Check sheet for the modelled part. Datum: model origin and axes. Units: mm. Round coordinates to 2 decimals unless told otherwise and drop trailing zeros. Write each loop counter-clockwise with the first axis right and the second up, starting at its lowest first coordinate (ties: lowest second). Pieces come first, ordered by that corner, then holes. Notation, with made-up numbers: (-18, 77) -> (11, 77) arc R32 cw to (11, 104) -> close; hole circle Ø1 at (29, 36.25). An arc over 180 degrees is marked (long way). Put each result on its own line as item: value. Start each with the question number.
from build123d import *

# Parameters (mm, degrees)
BOSS_EXTRUDE1_DEPTH     = 3.302
M3_CLEARANCE_HOLE1_D    = 3.4
SKETCH6_W               = 210.566
SKETCH6_H               = 3.302
BOSS_EXTRUDE3_DEPTH     = 1.62
SKETCH7_W               = 210.566
SKETCH7_H               = 3.302
BOSS_EXTRUDE4_DEPTH     = 5.18
M3_CLEARANCE_HOLE2_D    = 3.4
SKETCH21_R              = 20.32
CUT_EXTRUDE1_DEPTH      = 336.371396057
ADVANCEDHOLE1_OUTLINE_R = 1.6
ADVANCEDHOLE1_DEPTH     = 3.302
CUT_EXTRUDE2_REACH      = 337.371
SKETCH33_W              = 167.386
SKETCH33_H              = 21.59
FILLET1_R               = 6.35
CUT_EXTRUDE3_DEPTH      = 315.946962825
M5_CLEARANCE_HOLE1_D    = 5.5
M3_CLEARANCE_HOLE3_D    = 3.4
SKETCH40_W              = 22
SKETCH40_H              = 75
CUT_EXTRUDE4_DEPTH      = 315.946962825
FILLET2_R               = 3.81
FILLET3_R               = 2.032


# Read off the part's stored shape, not the designer's step: AdvancedHole1
with BuildPart() as part:
    # Sketch1 → Boss-Extrude1 (new body)
    with BuildSketch(Plane(origin=(0, 0, 0), x_dir=(1, 0, 0), z_dir=(0, 1, 0))):
        Polygon((105.283, -80.01), (105.283, 101.6), (-105.283, 101.6), (-105.283, -80.01), (-83.693, -80.01), (-83.693, -101.6), (83.693, -101.6), (83.693, -80.01), align=None)
    extrude(amount=BOSS_EXTRUDE1_DEPTH)

    # M3 Clearance Hole1 (through all)
    with Locations(Plane(origin=(0, 3.302, 0), x_dir=(1, 0, 0), z_dir=(0, 1, 0))):
        with Locations((-95.377, -54.61), (-95.377, 57.15), (95.377, 57.15), (95.377, -54.61)):
            Hole(M3_CLEARANCE_HOLE1_D / 2)

    # Sketch6 → Boss-Extrude3 (add)
    with BuildSketch(Plane(origin=(0, 0, -101.6), x_dir=(-1, 0, 0), z_dir=(0, 0, -1))):
        with Locations((0, 1.651)):
            Rectangle(SKETCH6_W, SKETCH6_H)
    extrude(amount=BOSS_EXTRUDE3_DEPTH)

    # Sketch7 → Boss-Extrude4 (add)
    with BuildSketch(Plane(origin=(0, 0, -103.22), x_dir=(-1, 0, 0), z_dir=(0, 0, -1))):
        with Locations((0, 1.651)):
            Rectangle(SKETCH7_W, SKETCH7_H)
    extrude(amount=BOSS_EXTRUDE4_DEPTH)


with BuildPart() as body_2:
    # Mirror2: mirrored copy
    add(part.part.mirror(Plane(origin=(0, 0, -108.4), x_dir=(1, 0, 0), z_dir=(0, 0, -1))))


with BuildPart() as part_1:
    add(part.part)

    # Combine1: union body 2
    add(body_2.part)

    # M3 Clearance Hole2 (through all)
    with Locations(Plane(origin=(0, 3.302, 0), x_dir=(1, 0, 0), z_dir=(0, 1, 0))):
        with Locations((-58.293, -91.6), (58.293, -91.6), (-58.293, 308.4), (58.293, 308.4)):
            Hole(M3_CLEARANCE_HOLE2_D / 2)

    # Sketch21 → Cut-Extrude1 (cut, through all)
    with BuildSketch(Plane(origin=(0, 3.302, 0), x_dir=(1, 0, 0), z_dir=(0, 1, 0))):
        with Locations(Location((0, 108.4, 0), (0, 0, 270))):
            Circle(SKETCH21_R)
    extrude(amount=-CUT_EXTRUDE1_DEPTH, mode=Mode.SUBTRACT)

    # AdvancedHole1 outline → AdvancedHole1 (cut)
    with BuildSketch(Plane(origin=(0, 0, 0), x_dir=(1, 0, 0), z_dir=(0, 1, 0))):
        with Locations((-11.624680448, 199.4)):
            Circle(ADVANCEDHOLE1_OUTLINE_R)
        with Locations((-18.809128073, 177.28854382)):
            Circle(ADVANCEDHOLE1_OUTLINE_R)
        with Locations((0, 163.62291236)):
            Circle(ADVANCEDHOLE1_OUTLINE_R)
        with Locations((18.809128073, 177.28854382)):
            Circle(ADVANCEDHOLE1_OUTLINE_R)
        with Locations((11.624680448, 199.4)):
            Circle(ADVANCEDHOLE1_OUTLINE_R)
    extrude(amount=ADVANCEDHOLE1_DEPTH, mode=Mode.SUBTRACT)

    # Sketch33 → Cut-Extrude2 (cut, up to next)
    with BuildSketch(Plane(origin=(0, 3.302, 0), x_dir=(1, 0, 0), z_dir=(0, 1, 0)), mode=Mode.PRIVATE) as cut_extrude2_sk1:
        with Locations((0, 307.605)):
            Rectangle(SKETCH33_W, SKETCH33_H)
    cut_extrude2_tool1 = extrude(cut_extrude2_sk1.sketch, amount=-CUT_EXTRUDE2_REACH, mode=Mode.PRIVATE) & part_1.part
    # Sketch33 → Cut-Extrude2 (cut, up to next)
    with BuildSketch(Plane(origin=(0, 3.302, 0), x_dir=(1, 0, 0), z_dir=(0, 1, 0)), mode=Mode.PRIVATE) as cut_extrude2_sk2:
        with Locations((0, -90.805)):
            Rectangle(SKETCH33_W, SKETCH33_H)
    cut_extrude2_tool2 = extrude(cut_extrude2_sk2.sketch, amount=-CUT_EXTRUDE2_REACH, mode=Mode.PRIVATE) & part_1.part
    add(cut_extrude2_tool1.solids().sort_by_distance((0, 3.302, -307.605))[0], mode=Mode.SUBTRACT)
    add(cut_extrude2_tool2.solids().sort_by_distance((0, 3.302, 90.805))[0], mode=Mode.SUBTRACT)

    # Fillet1
    fillet1_edges = [part_1.edges().sort_by_distance(p)[0] for p in [
        (-105.283, 1.651, 80.01),
        (105.283, 1.651, 80.01),
        (105.283, 1.651, -296.81),
        (-105.283, 1.651, -296.81),
    ]]
    fillet(fillet1_edges, radius=FILLET1_R)

    # Sketch24 → Cut-Extrude3 (cut, through all)
    with BuildSketch(Plane(origin=(0, 3.302, 0), x_dir=(1, 0, 0), z_dir=(0, 1, 0))):
        with BuildLine():
            Line((68.288075685, -5.771611822), (70.099809001, -12.533092606))
            ThreePointArc((70.099809001, -12.533092606), (69.039148829, -14.370209913), (67.202031522, -13.309549741))
            Line((67.202031522, -13.309549741), (65.390298207, -6.548068957))
            ThreePointArc((65.390298207, -6.548068957), (66.450958378, -4.71095165), (68.288075685, -5.771611822))
        make_face()
        with BuildLine():
            Line((76.311466084, -35.715312437), (78.123199399, -42.476793221))
            ThreePointArc((78.123199399, -42.476793221), (77.062539228, -44.313910528), (75.22542192, -43.253250356))
            Line((75.22542192, -43.253250356), (73.413688605, -36.491769572))
            ThreePointArc((73.413688605, -36.491769572), (74.474348777, -34.654652265), (76.311466084, -35.715312437))
        make_face()
        with BuildLine():
            Line((38.34437507, -13.79500222), (40.156108386, -20.556483004))
            ThreePointArc((40.156108386, -20.556483004), (39.095448214, -22.393600311), (37.258330907, -21.332940139))
            Line((37.258330907, -21.332940139), (35.446597592, -14.571459355))
            ThreePointArc((35.446597592, -14.571459355), (36.507257763, -12.734342048), (38.34437507, -13.79500222))
        make_face()
        with BuildLine():
            Line((46.367765469, -43.738702835), (48.179498784, -50.500183619))
            ThreePointArc((48.179498784, -50.500183619), (47.118838613, -52.337300926), (45.281721306, -51.276640754))
            Line((45.281721306, -51.276640754), (43.46998799, -44.51515997))
            ThreePointArc((43.46998799, -44.51515997), (44.530648162, -42.678042663), (46.367765469, -43.738702835))
        make_face()
    extrude(amount=-CUT_EXTRUDE3_DEPTH, mode=Mode.SUBTRACT)

    # M5 Clearance Hole1 (through all)
    with Locations(Plane(origin=(0, 3.302, 0), x_dir=(1, 0, 0), z_dir=(0, 1, 0))):
        with Locations((42.731024346, 23.92564608)):
            Hole(M5_CLEARANCE_HOLE1_D / 2)

    # M3 Clearance Hole3 (through all)
    with Locations(Plane(origin=(0, 3.302, 0), x_dir=(1, 0, 0), z_dir=(0, 1, 0))):
        with Locations((9.017, 19.05), (14.097, -29.21), (-67.183, 19.05), (-67.183, -29.21)):
            Hole(M3_CLEARANCE_HOLE3_D / 2)

    # Sketch40 → Cut-Extrude4 (cut, through all)
    with BuildSketch(Plane(origin=(0, 3.302, 0), x_dir=(1, 0, 0), z_dir=(0, 1, 0))):
        with Locations((94.283, 108.4)):
            Rectangle(SKETCH40_W, SKETCH40_H)
    extrude(amount=-CUT_EXTRUDE4_DEPTH, mode=Mode.SUBTRACT)

    # Fillet2
    fillet2_edges = [part_1.edges().sort_by_distance(p)[0] for p in [
        (105.283, 1.651, -145.9),
        (105.283, 1.651, -70.9),
    ]]
    fillet(fillet2_edges, radius=FILLET2_R)

    # Fillet3
    fillet3_edges = [part_1.edges().sort_by_distance(p)[0] for p in [
        (83.283, 1.651, -70.9),
        (83.283, 1.651, -145.9),
    ]]
    fillet(fillet3_edges, radius=FILLET3_R)


solid = part_1.part
1. Material ranges on L1, parallel to X at y = 1.5, z = 29.21; L2, parallel to Z at x = 95, y = 0.3; L3, parallel to X at y = 1.4, z = -57.15, recorded low to high. Write a range as [from, to].
2. Section check B-B, the plane y = 0.85. Give the number of separate pieces and of enclosed holes in the cut face, then the cut area to 3 significant figures.
3. Gauge pin test, flat end, axial feed: P1, Ø2.5, axis at x = 14.097, z = 29.21, coming from the +Y side. Record the tip position at first contact, or that the pin passes through.
4. Section check A-A, the plane z = -101.5. Enter the section's corners in (x, y), then the cut area to 3 significant figures.
5. Draft check along Z on faces 1 (the cylindrical face through (6.104, 1.674, -89.018)), 2 (the flat face through (-22, 3.302, -111)). Enter one of: released by +Z, released by -Z, zero draft, split by the parting line, or undercut.
Reply:
1. L1: x = [-105.28, -68.88], [-65.48, 12.4], [15.8, 105.28]
1. L2: z = [-296.81, -273.07], [-269.75, -161.31], [-157.99, -145.9], [-70.9, -58.81], [-55.49, 52.95], [56.27, 80.01]
1. L3: x = [-105.28, -97.08], [-93.68, 93.68], [97.08, 105.28]
2. separate pieces: 1
2. enclosed holes: 23
2. area: 76,100 mm2
3. P1: passes through
4. outline: (-105.28, 0) -> (-19.11, 0) -> (-19.11, 3.3) -> (-105.28, 3.3) -> close; (19.11, 0) -> (83.28, 0) -> (83.28, 3.3) -> (19.11, 3.3) -> close
4. area: 496 mm2
5. face 1: undercut
5. face 2: zero draft
